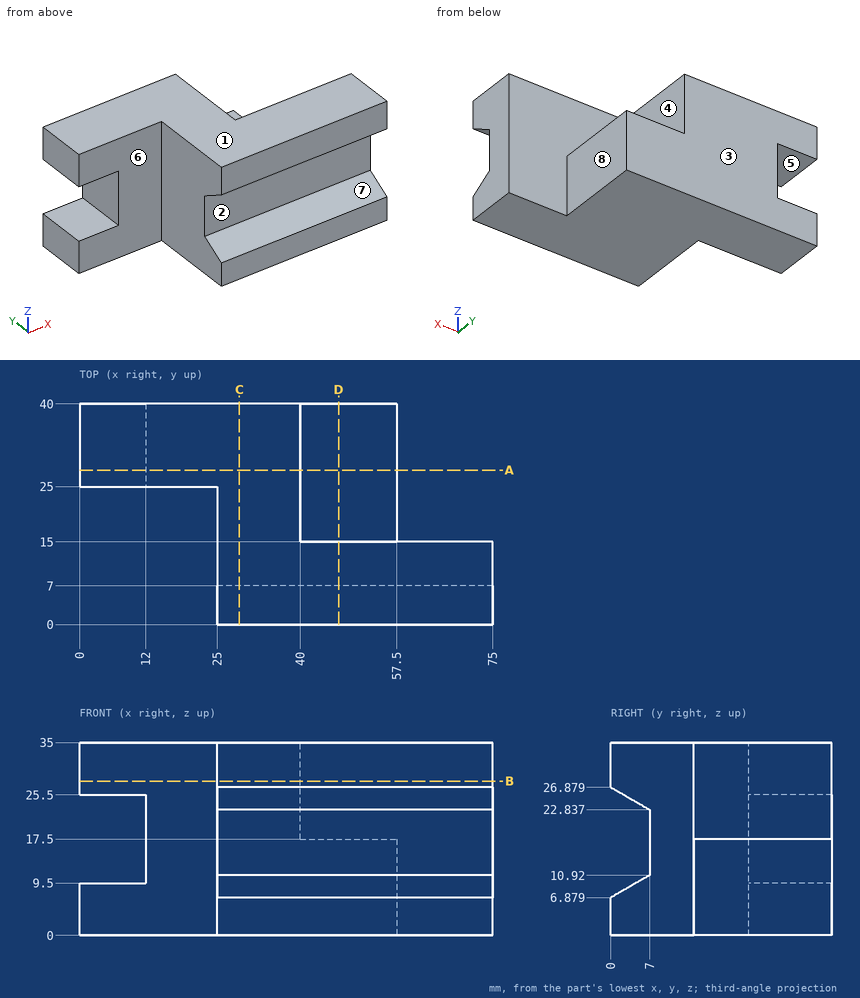
Verification items for this drawing (mm, ordinates from the low corner). A direction names the side the tool comes from. Give positions to 0.01 mm unless a question says otherwise; leave off trailing zeros. Loops run counter-clockwise (first coordinate to the right, second up) from the corner with the lowest first, then second, coordinate; pieces in that order, holes last. Notation, with made-up numbers: M 83,-27.75 L 95,-27.75 A20 ccw 95,-10.75 Z; hole C 41,84.25 d9. An arc over 180 degrees is marked long. Return JSON: item names as keys, results as strings. Group by question number.
1. Cross-section at D-D on x = 47. Record the boundary of the cut face in (y, z).
2. Go/stop test with flat-tipped pins: pin 1 (7.5 mm diameter, centred on y = 31, z = 15.5, fed in from -X); pin 2 (5 mm diameter, centred on x = 45, y = 25, fed in from +Z); pin 3 (5 mm diameter, centred on y = 6, z = 21.5, fed in from -X); pin 4 (3.5 mm diameter, centred on x = 5, y = 33.5, fed in from -Z). Record where each tip stops, or that it passes through.
3. Cross-section at A-A on y = 28. Record the boundary of the cut face in (x, z).
4. Cross-section at B-B on z = 28. Record the boundary of the cut face in (x, y).
5. Tool access check on the marked faces 4, 5, 6, 7 and 8. Record the directions out of +Z, -Z, +X, -X, +Y, -Y that give a thin tool (end or side, any length) a straight path to the whole face; none if there is none.
6. Thickness scan on L1, parallel to Z at x = 42, y = 17.5; L2, parallel to Y at x = 57, z = 20; L3, parallel to Y at x = 12.5, z = 14. Record the ranges inside material, lowest first.
7. Mould release check, pull along Z, two halves, no side actions. Record for the marked faces 1, 2 and 3: released by +Z, released by -Z, zero draft, split by the parting line, or undercut.
8. Cross-section at C-C on x = 29. Record the boundary of the cut face in (y, z).
Return value:
{
 "1": {"outline": "M 0,0 L 40,0 L 40,17.5 L 15,17.5 L 15,35 L 0,35 L 0,26.88 L 7,22.84 L 7,10.92 L 0,6.88 Z"},
 "2": {"pin 1": "x = 12", "pin 2": "z = 17.5", "pin 3": "x = 25", "pin 4": "z = 0"},
 "3": {"outline": "M 0,0 L 57.5,0 L 57.5,17.5 L 40,17.5 L 40,35 L 0,35 L 0,25.5 L 12,25.5 L 12,9.5 L 0,9.5 Z"},
 "4": {"outline": "M 0,25 L 25,25 L 25,0 L 75,0 L 75,15 L 40,15 L 40,40 L 0,40 Z"},
 "5": {"face 4": "+Z, +X, +Y", "face 5": "-X, +Y, -Y", "face 6": "+Z, -Z, -X, -Y", "face 7": "+X, -X, -Y", "face 8": "+Z, -Z, +X, +Y"},
 "6": {"L1": "0 to 17.5", "L2": "7 to 15", "L3": "25 to 40"},
 "7": {"face 1": "released by +Z", "face 2": "undercut", "face 3": "zero draft"},
 "8": {"outline": "M 0,0 L 40,0 L 40,35 L 0,35 L 0,26.88 L 7,22.84 L 7,10.92 L 0,6.88 Z"}
}
